Autodesk Inventor part; units mm, degrees
ref_plane "YZ Plane" through (0, 0, 0) normal (1, 0, 0) x (0, 1, 0)
ref_plane "XZ Plane" through (0, 0, 0) normal (0, 1, 0) x (-1, 0, 0)
ref_plane "XY Plane" through (0, 0, 0) normal (0, 0, 1) x (1, 0, 0)
sketch "Sketch1" plane through (0, 0, 0) normal (0, 1, 0) x (-1, 0, 0)
  line L0 (61.9125, -76.2) -> (-61.9125, -76.2)
  line L1 (-61.9125, -76.2) -> (-61.9125, 76.2)
  line L2 (-61.9125, 76.2) -> (61.9125, 76.2)
  line L3 (61.9125, 76.2) -> (61.9125, -76.2)
  line L4 (61.9125, -76.2) -> (-61.9125, 76.2) construction
  line L5 (-61.9125, -76.2) -> (61.9125, 76.2) construction
  point P0 (0, 0)
  dimension "d0" = 152.4
  dimension "d1" = 123.825
extrude "Plate1" add sketch "Sketch1" along normal mid plane 3.175
sketch "Sketch3" plane through (58.7375, 1.5875, 76.2) normal (1, 0, 0) x (0, 1, 0)
  line L0 (0, -152.4) -> (0, 0)
  line L1 (0, 0) -> (-76.2, 0)
  line L2 (-76.2, 0) -> (-76.2, -152.4)
  line L3 (-76.2, -152.4) -> (0, -152.4)
edge flange "Flange1" height 76.2 angle 90 thickness 3.175 bend radius 3.175 thickness toward (1, 0, 0) relief tear relief width 3.175 relief depth 1.5875 corner gap 3.175 corner form 0 edges at (61.9125, -1.5875, 0) (-61.9125, -1.5875, 0) wall of the first edge with corners at (58.7375, 1.5875, -76.2) (58.7375, 1.5875, 76.2) (58.7375, -74.6125, 76.2) (58.7375, -74.6125, -76.2)
bend "Bend1"
corner "Corner1"
sketch "Sketch4" plane through (61.9125, -74.6125, 76.2) normal (1, 0, 0) x (0, 0, -1)
  line L0 (0, 76.2) -> (152.4, 76.2) construction
  line L1 (0, 0) -> (0, 69.85) construction
  line L2 (41.7068, 44.45) -> (110.6932, 44.45) construction
  point P0 (76.2, 74.6125)
  point P1 (76.2, 44.45)
  point P2 (76.2, 76.2)
  dimension "d14" = 31.75
  dimension "d15" = 68.9864
hole "Hole1" at (61.9125, -30.1625, 34.4932) at (61.9125, -30.1625, -34.4932) direction (-1, 0, 0) diameter 25.4 end through all
sketch "Sketch5" plane through (0, 1.5875, 0) normal (0, 1, 0) x (1, 0, 0)
  circle A0 centre (0, 0) radius 31.75 construction
  point P0 (0, 31.75)
  dimension "d24" = 63.5
hole "Hole2" at (0, 1.5875, -31.75) direction (0, -1, 0) diameter 5.1054 end through all
pattern_circular "Circular Pattern1" count 6 over 360 about axis through (0, -10, 0) along (0, 1, 0) of "Hole2"
sketch "Sketch6" plane through (61.9125, -74.6125, 76.2) normal (1, 0, 0) x (0, 0, -1)
  line L0 (19.05, 12.7) -> (57.15, 12.7) construction
  line L1 (57.15, 12.7) -> (95.25, 12.7) construction
  line L2 (95.25, 12.7) -> (133.35, 12.7) construction
  line L3 (152.4, 0) -> (0, 0)
  point P0 (76.2, 74.6125)
  point P1 (76.2, 12.7)
  point P2 (76.2, 0)
  dimension "d35" = 38.1
  dimension "d36" = 38.1
  dimension "d37" = 38.1
  dimension "d38" = 12.7
hole "Hole3" at (61.9125, -61.9125, 57.15) at (61.9125, -61.9125, 19.05) at (61.9125, -61.9125, -19.05) at (61.9125, -61.9125, -57.15) direction (-1, 0, 0) diameter 5.1054 end through all
sketch "Sketch7" plane through (61.9125, -74.6125, 76.2) normal (1, 0, 0) x (0, 0, -1)
  circle A0 centre (95.25, 12.7) radius 2.5527
  circle A1 centre (19.05, 12.7) radius 2.5527
  circle A2 centre (57.15, 12.7) radius 2.5527
  circle A3 centre (133.35, 12.7) radius 2.5527
  circle A4 centre (41.7068, 44.45) radius 12.7
  circle A5 centre (110.6932, 44.45) radius 12.7
  line L0 (0, 69.85) -> (152.4, 69.85)
  line L1 (152.4, 69.85) -> (152.4, 0)
  line L2 (152.4, 0) -> (0, 0)
  line L3 (0, 0) -> (0, 69.85)
  line L4 (20.6883, 44.45) -> (62.7253, 44.45) construction
  line L5 (89.6747, 44.45) -> (131.7117, 44.45) construction
  point P0 (76.2, 74.6125)
  dimension "d46" = 42.037
  dimension "d47" = 42.037
hole "Hole4" at (61.9125, -30.1625, 55.5117) at (61.9125, -30.1625, 13.4747) at (61.9125, -30.1625, -13.4747) at (61.9125, -30.1625, -55.5117) direction (-1, 0, 0) diameter 5.1054 end through all
equation "\"d22\" = Thickness"
equation "\"d30\" = Thickness"
equation "\"d36\" = d35"
equation "\"d37\" = d35"
equation "\"d44\" = Thickness"
equation "\"d47\" = d46"
equation "\"d53\" = Thickness"
equation "\"d2\" = Thickness"
equation "\"d4\" = BendReliefWidth"
equation "\"d5\" = BendReliefDepth"
equation "\"d6\" = MinimumRemnant"
equation "\"d7\" = TransitionRadius"
equation "\"d10\" = BendRadius"
equation "\"d11\" = CornerReliefSize"
equation "\"d12\" = GapSize"
equation "\"d13\" = JacobiRadiusSize"
equation "\"BendRadius\" = Thickness"
equation "\"BendReliefWidth\" = Thickness"
equation "\"BendReliefDepth\" = 0.5 * Thickness"
equation "\"CornerReliefSize\" = 4 * Thickness"
equation "\"MinimumRemnant\" = 2 * Thickness"
equation "\"TransitionRadius\" = BendRadius"
equation "\"JacobiRadiusSize\" = BendRadius"
equation "\"GapSize\" = Thickness"
properties part number "GP3-001" material "Aluminum 6061"
Source: CAD feature listing. Evaluate the final solid. Frame: model axes, mm. A direction names the side the tool comes from. Coordinates: 2 decimals unless noted, no trailing zeros. Loops run counter-clockwise (first coordinate to the right, second up) from the corner with the lowest first, then second, coordinate; pieces in that order, holes last. Notation, with made-up numbers: (77, 79) - (118, 79) arc R8 ccw to (118, 84) - close; hole circle Ø10 at (19, -25.5). An arc over 180 degrees is marked (long way). Return JSON: item names as keys, results as strings.
Q1. Section A-A, the plane y = -52.5. Return loops of the section in (x, z), plus the area to 3 significant figures.
Results:
{"outline": "(-61.91, -76.2) - (-58.74, -76.2) - (-58.74, 76.2) - (-61.91, 76.2) - close; (58.74, -76.2) - (61.91, -76.2) - (61.91, 76.2) - (58.74, 76.2) - close", "area": "968 mm2"}
Q2. Mould query, pull axis X, two halves, no side actions, for faces 3 (the cylindrical face through (25.94, -0.02, -13.85)), 4 (the cylindrical face through (-60.1, -0.32, -1.07)), 5 (the cylindrical face through (25.771, -0.022, 13.994)), 6 (the flat face through (60, -74.612, 1)). Classes: released by +X, released by -X, zero draft, split by the parting line, or undercut.
Results:
{"face 3": "undercut", "face 4": "released by -X", "face 5": "undercut", "face 6": "zero draft"}
Q3. Section B-B, the plane x = 0. Return loops of the section in (y, z).
Results:
{"outline": "(-1.59, -76.2) - (1.59, -76.2) - (1.59, -34.3) - (-1.59, -34.3) - close; (-1.59, -29.2) - (1.59, -29.2) - (1.59, 29.2) - (-1.59, 29.2) - close; (-1.59, 34.3) - (1.59, 34.3) - (1.59, 76.2) - (-1.59, 76.2) - close"}
Q4. Material intervals for line 1 along X through (y, z) = (-56.5, 65); line 2 along Y through (x, z) = (61.15, 57.15); line 3 along Y through (x, z) = (-3.5, -50), sorted ascending.
Results:
{"line 1": "-61.91 to -58.74, 58.74 to 61.91", "line 2": "-74.61 to -64.47, -59.36 to -32.12, -28.2 to -1.75", "line 3": "-1.59 to 1.59"}
Q5. Access query for faces 1 (the cylindrical face through (-60.347, -62.679, 54.715)), 2 (the cylindrical face through (57.83, -2.54, 1.07)). Directions: +Z, -Z, +X, -X, +Y, -Y. A direction counts if a zero-diameter tool reaches every point of the face in a straight line with its end or side. Return the directions, or none.
Results:
{"face 1": "+X, -X", "face 2": "+Z, -Z, -Y"}
Q6. Section C-C, the plane z = -31.75. Give the number of separate pieces and of enclosed holes in the cut face, plus the area to 3 significant figures.
Results:
{"separate pieces": "4", "enclosed holes": "0", "area": "670 mm2"}
Q7. Contact query for a flat-ended pin moving along its axis: P1, Ø8, axis at x = -27.5, z = 15.88, coming from the -Y side. Output: stop coordinate, or through.
Results:
{"P1": "y = -1.59"}
